from build123d import *

# Parameters (mm, degrees)
F0_R     = 15
F0_W     = 45
F0_H     = 15
F0_W_2   = 15
F1_DEPTH = 37.5
F2_SIZE  = 15
F4_DEPTH = 15
F5_D     = 20
F5_DEPTH = 15.001
F7_D     = 10


with BuildPart() as f1:
    # F0 (on Front) → F1 (new body, symmetric)
    with BuildSketch(Plane.XZ):
        with BuildLine():
            Line((-25, -25), (0, -25))
            ThreePointArc((0, -25), (17.6776695297, -17.6776695297), (25, 0))
            Line((25, 0), (25, 10))
            Line((25, 10), (25, 25))
            Line((25, 25), (0, 25))
            ThreePointArc((0, 25), (-17.6776695297, 17.6776695297), (-25, 0))
            Line((-25, 0), (-25, -10))
            Line((-25, -10), (-25, -25))
        make_face()
        Circle(F0_R, mode=Mode.SUBTRACT)
        Polygon((-50, -25), (-25, -25), (-25, -10), (-35, -10), (-35, 35), (-50, 35), align=None)
        with Locations((47.5, 17.5)):
            Rectangle(F0_W, F0_H)
        with Locations((-42.5, 42.5)):
            Rectangle(F0_W_2, F0_H)
    extrude(amount=F1_DEPTH, both=True)

    # F2
    f2_edges = [f1.edges().sort_by_distance(p)[0] for p in [
        (-42.5, -37.5, 50),
        (-42.5, 37.5, 50),
    ]]
    chamfer(f2_edges, length=F2_SIZE)

    # F3 (on face) → F4 (join, through all)
    with BuildSketch(Plane.YZ.offset(-35)):
        with BuildLine():
            ThreePointArc((-12.5, 15), (-2.5, 5), (7.5, 15))
            ThreePointArc((7.5, 15), (4.5710678119, 22.0710678119), (-2.5, 25))
            Line((-2.5, 25), (-2.5, 15))
            Line((-2.5, 15), (-12.5, 15))
        make_face()
    extrude(amount=-F4_DEPTH)

    # F5 (through all, one way)
    with BuildSketch(Plane.YZ.offset(-35)):
        with Locations((-2.5, 15)):
            Circle(F5_D / 2)
    extrude(amount=-F5_DEPTH, mode=Mode.SUBTRACT)

    # F7 (through all)
    with Locations(Plane.XY.offset(25)):
        with Locations((55, -17.5), (55, 17.5)):
            Hole(F7_D / 2)


solid = f1.part
The listing builds one solid part. Answer for the finished solid, in the listing's coordinates (mm). A direction names the side the tool comes from. Round coordinates to 2 decimals unless told otherwise and drop trailing zeros. Order: outer loops, then holes, each group sorted by start corner. A loop starts at its lowest first (then second) coordinate and runs counter-clockwise, first axis right, second up. Notation, with made-up numbers: (63.5, 38.5) -> (110.5, 38.5) arc R9 ccw to (110.5, 42.5) -> close; hole circle Ø8 at (-35, -3). An arc over 180 degrees is marked (long way). Write each question's results on one line, items separated by ' | '. Start each with the question number.
Q1. Each of these flat-tipped pins is pushed along its axis until it touches: pin 1 (8 mm diameter, centred on y = 9.5, z = 5, fed in from +X); pin 2 (1.5 mm diameter, centred on x = -12, z = 5.5, fed in from -Y); pin 3 (18 mm diameter, centred on y = -2.5, z = 15, fed in from -X); pin 4 (21 mm diameter, centred on x = 18.5, y = -10, fed in from +Z). Where does it stop, or does it pass through?
Q2. Find section C-C (y = 24). Determine the outline of the cut face in (x, z), then the cut area to 3 significant figures.
Q3. Which of the six approach directions +Z, -Z, +X, -X, +Y, -Y give full straight-line access (tool end or side, diameter ignored) to faces 1 (the flat face through (-30, -1, -10)), 2 (the flat face through (25, -1, 5)), 3 (the flat face through (-43, 0, 50)), 4 (the cylindrical face through (-42.4, -9.87, 21.76)), 5 (the flat face through (35, -1, 25))?
Q4. Find section B-B (x = 55). Determine the outline of the cut face in (y, z).
Q5. Find section D-D (z = 6.5). Determine the outline of the cut face in (x, y), then the cut area to 3 significant figures.
Q6. The mould has two halves that part along Y. Classify faces 6 (the flat face through (-18, -37.5, 5)), 7 (the flat face through (47, -1, 10)), 8 (the cylindrical face through (59, -20.5, 17.4)), 9 (the flat face through (-42.6, 30.1, 42.4)): pulls with the +Y half, pulls with the -Y half, needs draft (parallel to the pull), parting line crosses it, or undercut.
Q7. Find section A-A (y = -2.5). Determine the outline of the cut face in (x, z), then the cut area to 3 significant figures.
Q8. Straight lines are drawn through the part: probe 1 along Y at (x, z) = (55, 18); probe 2 along X at (y, z) = (-23, 9); probe 3 along X at (y, z) = (12.5, 4.5). For each, find the intervals that lie inside material, in ascending order. Write a range as from..to.
Worked answers:
1) pin 1: stops at x = 25 | pin 2: passes through | pin 3: stops at x = -24.27 | pin 4: stops at z = 25
2) outline: (-50, -25) -> (0, -25) arc R25 ccw to (25, 0) -> (25, 10) -> (70, 10) -> (70, 25) -> (0, 25) arc R25 ccw to (-25, 0) -> (-25, -10) -> (-35, -10) -> (-35, 48.5) -> (-50, 48.5) -> close; hole circle Ø30 at (0, 0) | area: 3,450 mm2
3) face 1: +Z, +Y, -Y | face 2: -Z, +X, +Y, -Y | face 3: +Z, +X, -X, +Y, -Y | face 4: -X | face 5: +Z, +X, +Y, -Y
4) outline: (-37.5, 10) -> (-22.5, 10) -> (-22.5, 25) -> (-37.5, 25) -> close; (-12.5, 10) -> (12.5, 10) -> (12.5, 25) -> (-12.5, 25) -> close; (22.5, 10) -> (37.5, 10) -> (37.5, 25) -> (22.5, 25) -> close
5) outline: (-50, -37.5) -> (-35, -37.5) -> (-35, -7.77) -> (-50, -7.77) -> close; (-50, 2.77) -> (-35, 2.77) -> (-35, 37.5) -> (-50, 37.5) -> close; (-24.14, -37.5) -> (-13.52, -37.5) -> (-13.52, 37.5) -> (-24.14, 37.5) -> close; (13.52, -37.5) -> (25, -37.5) -> (25, 37.5) -> (13.52, 37.5) -> close | area: 2,620 mm2
6) face 6: pulls with the -Y half | face 7: needs draft | face 8: undercut | face 9: pulls with the +Y half
7) outline: (-50, -25) -> (0, -25) arc R25 ccw to (25, 0) -> (25, 10) -> (70, 10) -> (70, 25) -> (0, 25) arc R25 ccw to (-25, 0) -> (-25, -10) -> (-35, -10) -> (-35, 5) -> (-50, 5) -> close; (-50, 25) -> (-35, 25) -> (-35, 50) -> (-50, 50) -> close; hole circle Ø30 at (0, 0) | area: 3,170 mm2
8) probe 1: y = -37.5..-22.5, -12.5..12.5, 22.5..37.5 | probe 2: x = -50..-35, -23.32..-12, 12..25 | probe 3: x = -50..-35, -24.59..-14.31, 14.31..25
